from build123d import *

# Parameters (mm, degrees)
SKETCH1_W           = 170
SKETCH1_H           = 106
BOSS_EXTRUDE1_DEPTH = 6
FILLET1_R           = 6
CUT_EXTRUDE1_DEPTH  = 4
CUT_EXTRUDE2_DEPTH  = 201.429538741
CUT_EXTRUDE3_DEPTH  = 25
CUT_EXTRUDE4_DEPTH  = 201.379639771
FILLET2_R           = 1


with BuildPart() as part:
    # Sketch1 → Boss-Extrude1 (new body)
    with BuildSketch(Plane(origin=(0, 0, 0), x_dir=(1, 0, 0), z_dir=(0, 1, 0))):
        with Locations((85, -53)):
            Rectangle(SKETCH1_W, SKETCH1_H)
    extrude(amount=BOSS_EXTRUDE1_DEPTH)

    # Fillet1
    fillet1_edges = [part.edges().sort_by_distance(p)[0] for p in [
        (85, 6, 106),
        (85, 6, 0),
    ]]
    fillet(fillet1_edges, radius=FILLET1_R - 0.0001)  # a hair under: the kernel refuses the full size

    # Sketch2 → Cut-Extrude1 (cut)
    with BuildSketch(Plane(origin=(0, 6, 0), x_dir=(1, 0, 0), z_dir=(0, 1, 0))):
        with BuildLine():
            Line((55, -13), (115, -13))
            ThreePointArc((115, -13), (155, -53), (115, -93))
            Line((115, -93), (55, -93))
            ThreePointArc((55, -93), (15, -53), (55, -13))
        make_face()
    extrude(amount=-CUT_EXTRUDE1_DEPTH, mode=Mode.SUBTRACT)

    # Sketch3 → Cut-Extrude2 (cut, through all)
    with BuildSketch(Plane(origin=(0, 6, 0), x_dir=(1, 0, 0), z_dir=(0, 1, 0))):
        with BuildLine():
            Line((2, -53), (2, -38))
            Line((2, -38), (17.919007565, -38))
            ThreePointArc((17.919007565, -38), (15, -53), (17.919007565, -68))
            Line((17.919007565, -68), (2, -68))
            Line((2, -68), (2, -53))
        make_face()
    extrude(amount=-CUT_EXTRUDE2_DEPTH, mode=Mode.SUBTRACT)

    # Sketch5 → Cut-Extrude3 (cut)
    with BuildSketch(Plane.XY):
        with BuildLine():
            Line((49, 6), (121, 6))
            ThreePointArc((121, 6), (118.171572875, 4.828427125), (117, 2))
            Line((117, 2), (53, 2))
            ThreePointArc((53, 2), (51.828427125, 4.828427125), (49, 6))
        make_face()
    extrude(amount=CUT_EXTRUDE3_DEPTH, mode=Mode.SUBTRACT)

    # Sketch8 → Cut-Extrude4 (cut, through all)
    with BuildSketch(Plane(origin=(0, 2, 0), x_dir=(1, 0, 0), z_dir=(0, 1, 0))):
        with BuildLine():
            Line((55, -18), (115, -18))
            ThreePointArc((115, -18), (150, -53), (115, -88))
            Line((115, -88), (55, -88))
            ThreePointArc((55, -88), (20, -53), (55, -18))
        make_face()
    extrude(amount=-CUT_EXTRUDE4_DEPTH, mode=Mode.SUBTRACT)

    # Fillet2
    fillet2_edges = [part.edges().sort_by_distance(p)[0] for p in [
        (2, 3, 38),
        (2, 3, 68),
    ]]
    fillet(fillet2_edges, radius=FILLET2_R)


solid = part.part
Can you work these out from the model? Positions are in its coordinate system, mm. A direction names the side the tool comes from. Give positions to 0.01 mm unless a question says otherwise; leave off trailing zeros. Order: outer loops, then holes, each group sorted by start corner. A loop starts at its lowest first (then second) coordinate and runs counter-clockwise, first axis right, second up. Notation, with made-up numbers: M 27,-19 L 54,-19 A33 ccw 54,13 Z; hole C 86.25,62.5 d11. An arc over 180 degrees is marked long. Use one line per item in the form item = value.
Item 1: For faces 4 (the flat face through (10, 3, 38)), 5 (the flat face through (85, 6, 95)), 6 (the flat face through (0, 3, 54)), 7 (the flat face through (85, 2, 16)), 8 (the cylindrical face through (118.203, 4.859, 8.263)), which set-ups out of +Z, -Z, +X, -X, +Y, -Y let a thin tool reach every point of the face, with its end or its side?
Values follow:
face_4 = +Y, -Y
face_5 = +Z, -Z, +X, -X, +Y
face_6 = +Z, -Z, -X, +Y, -Y
face_7 = +Y
face_8 = -Z, +Y
Item 2: If we section it at B-B, the plane z = 53: Write out the boundary of the cut face in (x, y), and give its area (3 significant figures).
Values follow:
outline = M 0,0 L 2,0 L 2,6 L 0,6 Z; M 15,0 L 20,0 L 20,2 L 15,2 Z; M 150,0 L 170,0 L 170,6 L 155,6 L 155,2 L 150,2 Z
area = 122 mm^2
Item 3: Thinking about a two-plate mould opening in X: for faces 1 (the flat face through (170, 3, 54)), 2 (the flat face through (84, 0, 17)), 3 (the cylindrical face through (32.916, 4.028, 86.351)), which applies, pulls with the +X half, pulls with the -X half, needs draft (parallel to the pull), parting line crosses it, or undercut?
Values follow:
face_1 = pulls with the +X half
face_2 = needs draft
face_3 = undercut
Item 4: If I drill on line 1 along X through (y, z) = (1.5, 56); line 2 along X through (y, z) = (1.5, 24.5); line 3 along X through (y, z) = (5, 89), over which ranges is the centre line in solid material (lowest first)? Write a range as [from, to].
Values follow:
line_1 = [0, 2], [15.11, 20.13], [149.87, 170]
line_2 = [0, 34.68], [135.32, 170]
line_3 = [0, 37.56], [132.44, 170]
Item 5: Will these pins go through, and if not, where does the flat tip stop? pin 1 Ø1.6 at (x, y) = (98.5, 0.5) entering from -Z; pin 2 Ø1.8 at (x, y) = (13.5, 3) entering from +Z; pin 3 Ø1 at (x, y) = (106.5, 4) entering from +Z; pin 4 Ø1 at (x, y) = (88, 1) entering from +Z.
Values follow:
pin_1 = 0
pin_2 = 105.62
pin_3 = 104.87
pin_4 = 105.98
Item 6: If we section it at C-C, the plane z = 84: Write out the boundary of the cut face in (x, y).
Values follow:
outline = M 0,0 L 38.75,0 L 38.75,2 L 29.72,2 L 29.72,6 L 0,6 Z; M 131.25,0 L 170,0 L 170,6 L 140.28,6 L 140.28,2 L 131.25,2 Z
